Read the model definition and answer for the solid it produces. Units are mm, in the model's axes. Face numbers are marked on the shaded views. A direction names the side the tool comes from. Give positions to 0.01 mm unless a question says otherwise; leave off trailing zeros. Loops run counter-clockwise (first coordinate to the right, second up) from the corner with the lowest first, then second, coordinate; pieces in that order, holes last.
(1) Find section A-A, the plane x = -10. Write down the section's boundary in (y, z).
(2) Straight lines are drawn through the part: probe 1 along Y at (x, z) = (-10, 1.9); probe 2 along Z at (x, y) = (-12.5, 2.75); probe 3 along X at (y, z) = (-7.5, 2.6). For each, find the intervals that lie inside material, in ascending order.
(3) Which of the six approach directions +Z, -Z, +X, -X, +Y, -Y give full straight-line access (tool end or side, diameter ignored) to the marked faces 1 and 2?
(4) Find section C-C, the plane y = 0. Write down the section's boundary in (x, z), then the cut area to 3 significant figures.
(5) Find section D-D, the plane z = 1.75. Write down the section's boundary in (x, y), then the cut area to 3 significant figures.
(6) Find section B-B, the plane z = 3.1. Write down the section's boundary in (x, y), then the cut area to 3 significant figures.
(7) Determine the mould class of the marked faces 3, 4 and 5 for opening direction X: pulls with the +X half, pulls with the -X half, needs draft (parallel to the pull), parting line crosses it, or undercut.
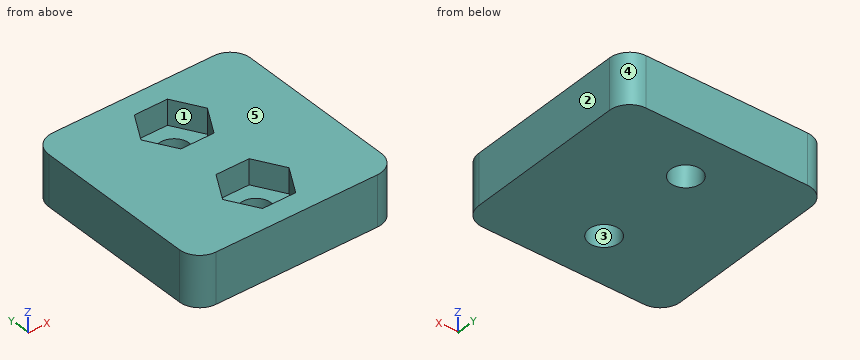
Autodesk Inventor part; units mm, degrees
ref_plane "YZ Plane" through (0, 0, 0) normal (1, 0, 0) x (0, 1, 0)
ref_plane "XZ Plane" through (0, 0, 0) normal (0, 1, 0) x (-1, 0, 0)
ref_plane "XY Plane" through (0, 0, 0) normal (0, 0, 1) x (1, 0, 0)
ref_plane "Work Plane1" through (0, 0, 0) normal (0, 0, 1) x (1, 0, 0)
sketch "Sketch1" plane through (0, 0, 0) normal (0, 0, 1) x (1, 0, 0)
  line L0 (7.4216, 7.4531) -> (-20, 7.4531)
  line L1 (-20, 7.4531) -> (-20, -9.4531)
  line L2 (20, -9.4531) -> (-20, -9.4531)
  line L3 (20, -4.1939) -> (20, -9.4531)
  line L4 (-20, 7.4531) -> (0, 7.4531)
  line L5 (0, 7.4531) -> (0, -12.5469)
  line L6 (0, -12.5469) -> (-20, -12.5469)
  line L7 (-20, -12.5469) -> (-20, 7.4531)
  arc A0 (8.8358, 6.8673) -> (7.4216, 7.4531) centre (7.4216, 5.4531) ccw
  arc A1 (19.5704, -3.8673) -> (20, -4.1939) centre (20.9847, -2.4531) ccw
  line L8 (8.8358, 6.8673) -> (19.5704, -3.8673)
  point P0 (0, 0)
  dimension "d0" = 20
  dimension "d1" = 20
extrude "Extrusion1" add sketch "Sketch1" along normal blind 5 contours L5 L2 L1 L0 | L5 L6 L7 L2
fillet "Fillet1" radius 2 4 edges at (0, 7.4531, 2.5) (0, -12.5469, 2.5) (-20, 7.4531, 2.5) (-20, -12.5469, 2.5)
sketch "Sketch2" plane through (0, 0, 5) normal (0, 0, 1) x (1, 0, 0)
  line L0 (-5.26, -4.4531) -> (-16.3573, -5.4531)
  arc A0 (-20, -10.5469) -> (-18, -12.5469) centre (-18, -10.5469) ccw
  line L1 (-18, -12.5469) -> (-2, -12.5469)
  arc A1 (-2, -12.5469) -> (0, -10.5469) centre (-2, -10.5469) ccw
  line L2 (0, -10.5469) -> (0, 5.4531)
  arc A2 (0, 5.4531) -> (-2, 7.4531) centre (-2, 5.4531) ccw
  line L3 (-2, 7.4531) -> (-18, 7.4531)
  arc A3 (-18, 7.4531) -> (-20, 5.4531) centre (-18, 5.4531) ccw
  line L4 (-20, 5.4531) -> (-20, -10.5469)
  line L5 (-10, -12.5469) -> (-10, 7.4531) construction
  line L6 (-2, 7.4531) -> (-18, 7.4531) construction
  line L7 (-10, -2.5469) -> (-10, 2.4531) construction
  line L8 (-10, 2.4531) -> (-10, -7.5469) construction
  point P0 (0, 0)
  dimension "d5" = 5
  dimension "d6" = 10
hole "Hole1" at (-10, 2.4531, 5) at (-10, -7.5469, 5) direction (0, 0, -1) diameter 3 end through all
sketch "Sketch3" plane through (0, 0, 5) normal (0, 0, 1) x (1, 0, 0)
  circle A0 centre (-10, 2.4531) radius 1.5
  circle A1 centre (-10, -7.5469) radius 1.5
  line L0 (-6.7091, 2.4531) -> (-8.3546, -0.3969)
  line L1 (-8.3546, -0.3969) -> (-11.6454, -0.3969)
  line L2 (-11.6454, -0.3969) -> (-13.2909, 2.4531)
  line L3 (-13.2909, 2.4531) -> (-11.6454, 5.3031)
  line L4 (-11.6454, 5.3031) -> (-8.3546, 5.3031)
  line L5 (-8.3546, 5.3031) -> (-6.7091, 2.4531)
  line L6 (-6.7091, -7.5469) -> (-8.3546, -10.3969)
  line L7 (-8.3546, -10.3969) -> (-11.6454, -10.3969)
  line L8 (-11.6454, -10.3969) -> (-13.2909, -7.5469)
  line L9 (-13.2909, -7.5469) -> (-11.6454, -4.6969)
  line L10 (-11.6454, -4.6969) -> (-8.3546, -4.6969)
  line L11 (-8.3546, -4.6969) -> (-6.7091, -7.5469)
  point P0 (0, 0)
  dimension "d14" = 5.7
extrude "Extrusion2" cut sketch "Sketch3" against normal blind 2.5
properties part number "little_holder"
Entries:
1. outline: (-12.55, 0) - (-9.05, 0) - (-9.05, 2.5) - (-10.4, 2.5) - (-10.4, 5) - (-12.55, 5) - close; (-6.05, 0) - (0.95, 0) - (0.95, 2.5) - (-0.4, 2.5) - (-0.4, 5) - (-4.7, 5) - (-4.7, 2.5) - (-6.05, 2.5) - close; (3.95, 0) - (7.45, 0) - (7.45, 5) - (5.3, 5) - (5.3, 2.5) - (3.95, 2.5) - close
2. probe 1: y = -12.55 to -9.05, -6.05 to 0.95, 3.95 to 7.45
2. probe 2: z = 0 to 2.5
2. probe 3: x = -20 to -13.26, -6.74 to 0
3. face 1: +Z
3. face 2: +Z, -Z, +X, +Y, -Y
4. outline: (-20, 0) - (0, 0) - (0, 5) - (-8.13, 5) - (-8.13, 2.5) - (-11.87, 2.5) - (-11.87, 5) - (-20, 5) - close
4. area: 90.6 mm2
5. outline: (-20, -10.55) arc R2 ccw to (-18, -12.55) - (-2, -12.55) arc R2 ccw to (0, -10.55) - (0, 5.45) arc R2 ccw to (-2, 7.45) - (-18, 7.45) arc R2 ccw to (-20, 5.45) - close; hole circle Ø3 at (-10, -7.55); hole circle Ø3 at (-10, 2.45)
5. area: 382 mm2
6. outline: (-20, -10.55) arc R2 ccw to (-18, -12.55) - (-2, -12.55) arc R2 ccw to (0, -10.55) - (0, 5.45) arc R2 ccw to (-2, 7.45) - (-18, 7.45) arc R2 ccw to (-20, 5.45) - close; hole (-13.29, -7.55) - (-11.65, -10.4) - (-8.35, -10.4) - (-6.71, -7.55) - (-8.35, -4.7) - (-11.65, -4.7) - close; hole (-13.29, 2.45) - (-11.65, -0.4) - (-8.35, -0.4) - (-6.71, 2.45) - (-8.35, 5.3) - (-11.65, 5.3) - close
6. area: 340 mm2
7. face 3: undercut
7. face 4: pulls with the +X half
7. face 5: needs draft
